Build history of the part. All positions in model axes, mm. Face numbers are marked on the shaded views. Give positions to 0.01 mm unless a question says otherwise; leave off trailing zeros. Loops run counter-clockwise (first coordinate to the right, second up) from the corner with the lowest first, then second, coordinate; pieces in that order, holes last. Notation, with made-up numbers: (-9, -4) -> (39, -4) arc R35 cw to (39, 30) -> close; hole circle Ø3 at (61, -16). An arc over 180 degrees is marked (long way). One line per question, with ' | ' between items. Start each with the question number.
(1) Slice it at C-C, the plane x = 2.6. Write the cut outline in (y, z).
(2) Flat gauge pins, fed straight in: pin 1 Ø2.5 at (y, z) = (-3.34, -4.06) entering from +X; pin 2 Ø2 at (x, y) = (2.5, -6.5) entering from -Z. Where does each tip first touch, or does it go through?
(3) Slice it at B-B, the plane z = -2.75. Write the cut outline in (x, y), then the cut area to 3 significant figures.
(4) Drill centre lines: L1, parallel to Z at x = 2.25, y = -5; L2, parallel to Y at x = 1.9, z = -2.75; L3, parallel to Y at x = 2.25, z = -3.7. Where is each one in solid material? Low to high. Write a range as from..to.
(5) Mould opens along Y. For the marked faces 1, 2, 3 and 4 say: pulls with the +Y half, pulls with the -Y half, needs draft (parallel to the pull), parting line crosses it, or undercut.
(6) Slice it at A-A, the plane y = -5. Write the cut outline in (x, z).
(7) Slice it at D-D, the plane y = -7. Write the cut outline in (x, z), then the cut area to 3 significant figures.
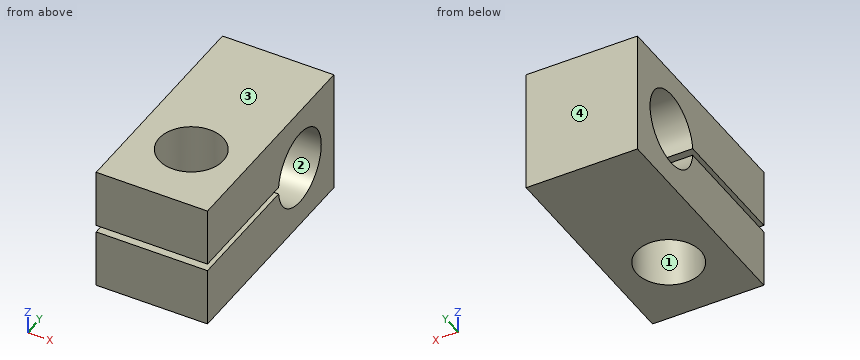
```python
from build123d import *

# Parameters (mm, degrees)
BOSS_EXTRUDE2_DEPTH = 4.5
SKETCH3_R           = 1.3
CUT_EXTRUDE1_DEPTH  = 10.5


with BuildPart() as part:
    # Sketch1 → Boss-Extrude2 (new body)
    with BuildSketch(Plane(origin=(0, 0, 0), x_dir=(0, 0, -1), z_dir=(1, 0, 0))):
        with BuildLine():
            Line((1.55613054, -9.91539795), (3.917713804, -9.916320319))
            Line((3.917713804, -9.916320319), (3.917713804, -4.855498596))
            ThreePointArc((3.917713804, -4.855498596), (4.062635704, -1.822441499), (4.208325788, -4.855461794))
            Line((4.208325788, -4.855461794), (4.208325788, -9.916433824))
            Line((4.208325788, -9.916433824), (6.579674081, -9.917360006))
            Line((6.579674081, -9.917360006), (6.579674081, -0.928463249))
            Line((6.579674081, -0.928463249), (1.55613054, -0.928463249))
            Line((1.55613054, -0.928463249), (1.55613054, -9.91539795))
        make_face()
    extrude(amount=BOSS_EXTRUDE2_DEPTH)

    # Sketch3 → Cut-Extrude1 (cut)
    with BuildSketch(Plane.XY.offset(-1.55613054)):
        with Locations((2.256029543, -7.121731935)):
            Circle(SKETCH3_R)
    extrude(amount=-CUT_EXTRUDE1_DEPTH, mode=Mode.SUBTRACT)


solid = part.part
```
Final values:
1) outline: (-9.92, -6.58) -> (-8.38, -6.58) -> (-8.38, -4.21) -> (-9.92, -4.21) -> close; (-9.92, -3.92) -> (-8.38, -3.92) -> (-8.38, -1.56) -> (-9.92, -1.56) -> close; (-5.87, -6.58) -> (-0.93, -6.58) -> (-0.93, -1.56) -> (-5.87, -1.56) -> (-5.87, -3.92) -> (-4.86, -3.92) arc R1.52 cw (long way) to (-4.86, -4.21) -> (-5.87, -4.21) -> close
2) pin 1: through | pin 2: z = -6.58
3) outline: (0, -9.92) -> (4.5, -9.92) -> (4.5, -4.11) -> (0, -4.11) -> close; (0, -2.58) -> (4.5, -2.58) -> (4.5, -0.93) -> (0, -0.93) -> close; hole circle Ø2.6 at (2.26, -7.12) | area: 28.2 mm2
4) L1: -6.58..-4.21, -3.92..-1.56 | L2: -9.92..-8.37, -5.87..-4.11, -2.58..-0.93 | L3: -9.92..-8.42, -5.82..-4.82, -1.87..-0.93
5) face 1: undercut | face 2: undercut | face 3: needs draft | face 4: pulls with the +Y half
6) outline: (0, -6.58) -> (4.5, -6.58) -> (4.5, -4.21) -> (0, -4.21) -> close; (0, -3.92) -> (4.5, -3.92) -> (4.5, -1.56) -> (0, -1.56) -> close
7) outline: (0, -6.58) -> (0.96, -6.58) -> (0.96, -4.21) -> (0, -4.21) -> close; (0, -3.92) -> (0.96, -3.92) -> (0.96, -1.56) -> (0, -1.56) -> close; (3.55, -6.58) -> (4.5, -6.58) -> (4.5, -4.21) -> (3.55, -4.21) -> close; (3.55, -3.92) -> (4.5, -3.92) -> (4.5, -1.56) -> (3.55, -1.56) -> close | area: 9.05 mm2
